Part model, mm, in its own coordinate system. A direction names the side the tool comes from. Round coordinates to 2 decimals unless told otherwise and drop trailing zeros. Loops run counter-clockwise (first coordinate to the right, second up) from the corner with the lowest first, then second, coordinate; pieces in that order, holes last.
(1) Cut at A-A on y = 0. List the corners of the cut face in (x, z), then the cut area to 3 significant figures.
(2) Flat gauge pins, fed straight in: pin 1 (4 mm diameter, centred on x = -1.5, z = -99, fed in from -Y); pin 2 (1.5 mm diameter, centred on x = -5.5, z = -95.5, fed in from -Y); pin 3 (1.5 mm diameter, centred on x = -6.5, z = -254.5, fed in from -Y); pin 4 (2 mm diameter, centred on y = 9, z = -114.5, fed in from +X). Where does each tip first touch, or does it go through?
(3) Probe probe 1 along Y at (x, z) = (0.75, 44); probe 2 along Z at (x, y) = (-9.75, 6.5); probe 3 along X at (y, z) = (-3, -41). List the from-to ranges inside material, lowest first.
(4) Cut at D-D on z = -78.5. List the corners of the cut face in (x, y).
(5) Cut at C-C on z = -162. List the corners of the cut face in (x, y).
(6) Tool access for faces 1 (the face through (2.17, -9.76, -223.95)), 2 (the face through (0.1, 10.2, 0)), 3 (the face through (0, 0, 80)): list every direction of +Z, -Z, +X, -X, +Y, -Y with a clear straight run to the whole face (end or side of a thin tool).
from build123d import *

# Parameters (mm, degrees)
CROQUIS1_R              = 10
SALIENTE_EXTRUIR1_DEPTH = 80
CROQUIS2_R              = 12.5
SALIENTE_EXTRUIR2_DEPTH = 150
CROQUIS3_R              = 10
SALIENTE_EXTRUIR3_DEPTH = 150


with BuildPart() as part:
    # Croquis1 → Saliente-Extruir1 (new body)
    with BuildSketch(Plane.XY):
        Circle(CROQUIS1_R)
    extrude(amount=SALIENTE_EXTRUIR1_DEPTH)

    # Croquis2 → Saliente-Extruir2 (add)
    with BuildSketch(Plane(origin=(0, 0, 0), x_dir=(-1, 0, 0), z_dir=(0, 0, -1))):
        Circle(CROQUIS2_R)
    extrude(amount=SALIENTE_EXTRUIR2_DEPTH)

    # Croquis3 → Saliente-Extruir3 (add)
    with BuildSketch(Plane(origin=(0, 0, -150), x_dir=(-1, 0, 0), z_dir=(0, 0, -1))):
        Circle(CROQUIS3_R)
    extrude(amount=SALIENTE_EXTRUIR3_DEPTH)


solid = part.part
Final values:
1. outline: (-12.5, -150) - (-10, -150) - (-10, -300) - (10, -300) - (10, -150) - (12.5, -150) - (12.5, 0) - (10, 0) - (10, 80) - (-10, 80) - (-10, 0) - (-12.5, 0) - close
1. area: 8,350 mm2
2. pin 1: stops at y = -12.5
2. pin 2: stops at y = -11.56
2. pin 3: stops at y = -8.18
2. pin 4: stops at x = 9.6
3. probe 1: y = -9.97 to 9.97
3. probe 2: z = -150 to 0
3. probe 3: x = -12.13 to 12.13
4. outline: circle Ø25 at (0, 0)
5. outline: circle Ø20 at (0, 0)
6. face 1: -Z
6. face 2: +Z
6. face 3: +Z, +X, -X, +Y, -Y
